```python
from build123d import *

# Parameters (mm, degrees)
SKETCH1_W           = 360
SKETCH1_H           = 30
BOSS_EXTRUDE1_DEPTH = 1.6
SKETCH2_W           = 10
SKETCH2_H           = 1.6
BOSS_EXTRUDE2_DEPTH = 1.6
CUT_EXTRUDE1_DEPTH  = 181.770904739
CUT_EXTRUDE2_DEPTH  = 181.770904739
SKETCH5_W           = 15
SKETCH5_H           = 30
CUT_EXTRUDE3_DEPTH  = 181.770904739
SKETCH6_W           = 4
SKETCH6_H           = 33.2
BOSS_EXTRUDE3_DEPTH = 1.6
FILLET1_R           = 4
BOSS_EXTRUDE4_DEPTH = 1.6
SKETCH8_R           = 1.6
CUT_EXTRUDE4_DEPTH  = 166.840646405


with BuildPart() as part:
    # Sketch1 → Boss-Extrude1 (new body)
    with BuildSketch(Plane.XY):
        Rectangle(SKETCH1_W, SKETCH1_H)
    extrude(amount=BOSS_EXTRUDE1_DEPTH)

    # Sketch2 → Boss-Extrude2 (add)
    with BuildSketch(Plane.XY.offset(1.6)):
        with Locations((120, 15.8)):
            Rectangle(SKETCH2_W, SKETCH2_H)
        with Locations((80, 15.8)):
            Rectangle(SKETCH2_W, SKETCH2_H)
        with Locations((160, 15.8)):
            Rectangle(SKETCH2_W, SKETCH2_H)
        with Locations((-160, 15.8)):
            Rectangle(SKETCH2_W, SKETCH2_H)
        with Locations((-120, 15.8)):
            Rectangle(SKETCH2_W, SKETCH2_H)
        with Locations((-80, 15.8)):
            Rectangle(SKETCH2_W, SKETCH2_H)
        with Locations((-120, -15.8)):
            Rectangle(SKETCH2_W, SKETCH2_H)
        with Locations((-80, -15.8)):
            Rectangle(SKETCH2_W, SKETCH2_H)
        with Locations((-160, -15.8)):
            Rectangle(SKETCH2_W, SKETCH2_H)
        with Locations((160, -15.8)):
            Rectangle(SKETCH2_W, SKETCH2_H)
        with Locations((120, -15.8)):
            Rectangle(SKETCH2_W, SKETCH2_H)
        with Locations((80, -15.8)):
            Rectangle(SKETCH2_W, SKETCH2_H)
    extrude(amount=-BOSS_EXTRUDE2_DEPTH)

    # Sketch3 → Cut-Extrude1 (cut, through all)
    with BuildSketch(Plane.XY.offset(1.6)):
        with BuildLine():
            Line((-167, 10), (-133, 10))
            ThreePointArc((-133, 10), (-132.076120467, 9.382683432), (-132.292893219, 8.292893219))
            Line((-132.292893219, 8.292893219), (-148.585786438, -8))
            ThreePointArc((-148.585786438, -8), (-150, -8.585786438), (-151.414213562, -8))
            Line((-151.414213562, -8), (-167.707106781, 8.292893219))
            ThreePointArc((-167.707106781, 8.292893219), (-167.923879533, 9.382683432), (-167, 10))
        make_face()
        with BuildLine():
            Line((-117, 10), (-83, 10))
            ThreePointArc((-83, 10), (-82.076120467, 9.382683432), (-82.292893219, 8.292893219))
            Line((-82.292893219, 8.292893219), (-98.585786438, -8))
            ThreePointArc((-98.585786438, -8), (-100, -8.585786438), (-101.414213562, -8))
            Line((-101.414213562, -8), (-117.707106781, 8.292893219))
            ThreePointArc((-117.707106781, 8.292893219), (-117.923879533, 9.382683432), (-117, 10))
        make_face()
        with BuildLine():
            Line((-67, 10), (-33, 10))
            ThreePointArc((-33, 10), (-32.076120467, 9.382683432), (-32.292893219, 8.292893219))
            Line((-32.292893219, 8.292893219), (-48.585786438, -8))
            ThreePointArc((-48.585786438, -8), (-50, -8.585786438), (-51.414213562, -8))
            Line((-51.414213562, -8), (-67.707106781, 8.292893219))
            ThreePointArc((-67.707106781, 8.292893219), (-67.923879533, 9.382683432), (-67, 10))
        make_face()
        with BuildLine():
            Line((-17, 10), (17, 10))
            ThreePointArc((17, 10), (17.923879533, 9.382683432), (17.707106781, 8.292893219))
            Line((17.707106781, 8.292893219), (1.414213562, -8))
            ThreePointArc((1.414213562, -8), (0, -8.585786438), (-1.414213562, -8))
            Line((-1.414213562, -8), (-17.707106781, 8.292893219))
            ThreePointArc((-17.707106781, 8.292893219), (-17.923879533, 9.382683432), (-17, 10))
        make_face()
        with BuildLine():
            Line((33, 10), (67, 10))
            ThreePointArc((67, 10), (67.923879533, 9.382683432), (67.707106781, 8.292893219))
            Line((67.707106781, 8.292893219), (51.414213562, -8))
            ThreePointArc((51.414213562, -8), (50, -8.585786438), (48.585786438, -8))
            Line((48.585786438, -8), (32.292893219, 8.292893219))
            ThreePointArc((32.292893219, 8.292893219), (32.076120467, 9.382683432), (33, 10))
        make_face()
        with BuildLine():
            Line((83, 10), (117, 10))
            ThreePointArc((117, 10), (117.923879533, 9.382683432), (117.707106781, 8.292893219))
            Line((117.707106781, 8.292893219), (101.414213562, -8))
            ThreePointArc((101.414213562, -8), (100, -8.585786438), (98.585786438, -8))
            Line((98.585786438, -8), (82.292893219, 8.292893219))
            ThreePointArc((82.292893219, 8.292893219), (82.076120467, 9.382683432), (83, 10))
        make_face()
        with BuildLine():
            Line((133, 10), (167, 10))
            ThreePointArc((167, 10), (167.923879533, 9.382683432), (167.707106781, 8.292893219))
            Line((167.707106781, 8.292893219), (151.414213562, -8))
            ThreePointArc((151.414213562, -8), (150, -8.585786438), (148.585786438, -8))
            Line((148.585786438, -8), (132.292893219, 8.292893219))
            ThreePointArc((132.292893219, 8.292893219), (132.076120467, 9.382683432), (133, 10))
        make_face()
    extrude(amount=-CUT_EXTRUDE1_DEPTH, mode=Mode.SUBTRACT)

    # Sketch4 → Cut-Extrude2 (cut, through all)
    with BuildSketch(Plane.XY.offset(1.6)):
        with BuildLine():
            Line((-143.414213562, -10), (-106.585786438, -10))
            ThreePointArc((-106.585786438, -10), (-105.661906905, -9.382683432), (-105.878679656, -8.292893219))
            Line((-105.878679656, -8.292893219), (-123.585786438, 9.414213562))
            ThreePointArc((-123.585786438, 9.414213562), (-125, 10), (-126.414213562, 9.414213562))
            Line((-126.414213562, 9.414213562), (-144.121320344, -8.292893219))
            ThreePointArc((-144.121320344, -8.292893219), (-144.338093095, -9.382683432), (-143.414213562, -10))
        make_face()
        with BuildLine():
            Line((-93.414213562, -10), (-56.585786438, -10))
            ThreePointArc((-56.585786438, -10), (-55.661906905, -9.382683432), (-55.878679656, -8.292893219))
            Line((-55.878679656, -8.292893219), (-73.585786438, 9.414213562))
            ThreePointArc((-73.585786438, 9.414213562), (-75, 10), (-76.414213562, 9.414213562))
            Line((-76.414213562, 9.414213562), (-94.121320344, -8.292893219))
            ThreePointArc((-94.121320344, -8.292893219), (-94.338093095, -9.382683432), (-93.414213562, -10))
        make_face()
        with BuildLine():
            Line((-43.414213562, -10), (-6.585786438, -10))
            ThreePointArc((-6.585786438, -10), (-5.661906905, -9.382683432), (-5.878679656, -8.292893219))
            Line((-5.878679656, -8.292893219), (-23.585786438, 9.414213562))
            ThreePointArc((-23.585786438, 9.414213562), (-25, 10), (-26.414213562, 9.414213562))
            Line((-26.414213562, 9.414213562), (-44.121320344, -8.292893219))
            ThreePointArc((-44.121320344, -8.292893219), (-44.338093095, -9.382683432), (-43.414213562, -10))
        make_face()
        with BuildLine():
            Line((6.585786438, -10), (43.414213562, -10))
            ThreePointArc((43.414213562, -10), (44.338093095, -9.382683432), (44.121320344, -8.292893219))
            Line((44.121320344, -8.292893219), (26.414213562, 9.414213562))
            ThreePointArc((26.414213562, 9.414213562), (25, 10), (23.585786438, 9.414213562))
            Line((23.585786438, 9.414213562), (5.878679656, -8.292893219))
            ThreePointArc((5.878679656, -8.292893219), (5.661906905, -9.382683432), (6.585786438, -10))
        make_face()
        with BuildLine():
            Line((56.585786438, -10), (93.414213562, -10))
            ThreePointArc((93.414213562, -10), (94.338093095, -9.382683432), (94.121320344, -8.292893219))
            Line((94.121320344, -8.292893219), (76.414213562, 9.414213562))
            ThreePointArc((76.414213562, 9.414213562), (75, 10), (73.585786438, 9.414213562))
            Line((73.585786438, 9.414213562), (55.878679656, -8.292893219))
            ThreePointArc((55.878679656, -8.292893219), (55.661906905, -9.382683432), (56.585786438, -10))
        make_face()
        with BuildLine():
            Line((106.585786438, -10), (143.414213562, -10))
            ThreePointArc((143.414213562, -10), (144.338093095, -9.382683432), (144.121320344, -8.292893219))
            Line((144.121320344, -8.292893219), (126.414213562, 9.414213562))
            ThreePointArc((126.414213562, 9.414213562), (125, 10), (123.585786438, 9.414213562))
            Line((123.585786438, 9.414213562), (105.878679656, -8.292893219))
            ThreePointArc((105.878679656, -8.292893219), (105.661906905, -9.382683432), (106.585786438, -10))
        make_face()
    extrude(amount=-CUT_EXTRUDE2_DEPTH, mode=Mode.SUBTRACT)

    # Sketch5 → Cut-Extrude3 (cut, through all)
    with BuildSketch(Plane.XY.offset(1.6)):
        with Locations((-172.5, 0)):
            Rectangle(SKETCH5_W, SKETCH5_H)
        with Locations((172.5, 0)):
            Rectangle(SKETCH5_W, SKETCH5_H)
    extrude(amount=-CUT_EXTRUDE3_DEPTH, mode=Mode.SUBTRACT)

    # Sketch6 → Boss-Extrude3 (add)
    with BuildSketch(Plane.XY.offset(1.6)):
        with Locations((-163, 0)):
            Rectangle(SKETCH6_W, SKETCH6_H)
        with Locations((163, 0)):
            Rectangle(SKETCH6_W, SKETCH6_H)
    extrude(amount=-BOSS_EXTRUDE3_DEPTH)

    # Fillet1
    fillet1_edges = [part.edges().sort_by_distance(p)[0] for p in [
        (-161, 10, 0.8),
        (-161, 1.585786438, 0.8),
        (161, 1.585786438, 0.8),
        (161, 10, 0.8),
    ]]
    fillet(fillet1_edges, radius=FILLET1_R)

    # Sketch7 → Boss-Extrude4 (add)
    with BuildSketch(Plane.XY.offset(1.6)):
        with BuildLine():
            Line((-26.414213562, 9.414213562), (-29.707106781, 6.121320344))
            ThreePointArc((-29.707106781, 6.121320344), (-28.733836735, 6.771638598), (-27.585786438, 7))
            Line((-27.585786438, 7), (-22.414213562, 7))
            ThreePointArc((-22.414213562, 7), (-21.266163265, 6.771638598), (-20.292893219, 6.121320344))
            Line((-20.292893219, 6.121320344), (-23.585786438, 9.414213562))
            ThreePointArc((-23.585786438, 9.414213562), (-25, 10), (-26.414213562, 9.414213562))
        make_face()
        with BuildLine():
            Line((23.585786438, 9.414213562), (20.292893219, 6.121320344))
            ThreePointArc((20.292893219, 6.121320344), (21.266163265, 6.771638598), (22.414213562, 7))
            Line((22.414213562, 7), (27.585786438, 7))
            ThreePointArc((27.585786438, 7), (28.733836735, 6.771638598), (29.707106781, 6.121320344))
            Line((29.707106781, 6.121320344), (26.414213562, 9.414213562))
            ThreePointArc((26.414213562, 9.414213562), (25, 10), (23.585786438, 9.414213562))
        make_face()
    extrude(amount=-BOSS_EXTRUDE4_DEPTH)

    # Sketch8 → Cut-Extrude4 (cut, through all)
    with BuildSketch(Plane.XY.offset(1.6)):
        with Locations((-25, 10)):
            Circle(SKETCH8_R)
        with Locations(Location((25, 10, 0), (0, 0, 180))):
            Circle(SKETCH8_R)
        with Locations((0, -12)):
            Circle(SKETCH8_R)
    extrude(amount=-CUT_EXTRUDE4_DEPTH, mode=Mode.SUBTRACT)


solid = part.part
```
Part model, mm, in its own coordinate system. A direction names the side the tool comes from. Round coordinates to 2 decimals unless told otherwise and drop trailing zeros. Loops run counter-clockwise (first coordinate to the right, second up) from the corner with the lowest first, then second, coordinate; pieces in that order, holes last.
Item 1: Mould opens along Y. For faces 3 (the face through (-64.61, 0.44, 0.81)), 4 (the face through (-2, -11, 1.6)) say: +Y half, -Y half, draft (parallel to the pull), parting line (faces both ways), or undercut.
Item 2: Drill centre lines: line 1 (Y direction, x = 25, z = 1.15); line 2 (Y direction, x = 0, z = 0.4); line 3 (Y direction, x = 149.5, z = 0.5). Where is each one in solid material? Low to high.
Item 3: Cut at B-B, the plane z = 0.4. State how many separate pieces and enclosed holes the cut face has, then the cut area to 3 significant figures.
Item 4: Drop flat-ended pins along their axis: P1, Ø1.5, axis at x = -73, y = 6.5, coming from the -Z side; P2, Ø0.8, axis at x = 127.5, z = 0.5, coming from the +Y side; P3, Ø0.5, axis at x = -144.5, z = 0.5, coming from the -Y side; P4, Ø1, axis at x = 74.5, y = -12, coming from the -Z side. Give the stop position or say it passes through.
Item 5: 3-axis set-ups, long thin cutter, end or side, ignore diameter. For faces 1 (the face through (37.02, -1.19, 0.81)), 2 (the face through (-2, -11, 0)): which of +Z, -Z, +X, -X, +Y, -Y reach the whole face in a straight line?
Item 6: Cut at A-A, the plane x = 110. Give the cut face in (y, z).
A:
1. face 3: undercut
1. face 4: draft
2. line 1: y = -15 to -10, 7 to 8.4, 11.6 to 15
2. line 2: y = -15 to -13.6, -10.4 to -8.59, 10 to 15
2. line 3: y = -15 to -8.52, 10 to 15
3. separate pieces: 1
3. enclosed holes: 16
3. area: 4,970 mm2
4. P1: passes through
4. P2: stops at y = 15
4. P3: stops at y = -15
4. P4: stops at z = 0
5. face 1: +Z, -Z
5. face 2: -Z, +X, -X, +Y, -Y
6. outline: (-15, 0) - (-10, 0) - (-10, 1.6) - (-15, 1.6) - close; (-4.17, 0) - (0.59, 0) - (0.59, 1.6) - (-4.17, 1.6) - close; (10, 0) - (15, 0) - (15, 1.6) - (10, 1.6) - close
